For this review, take the finished solid that the model builds, in its own axes (mm). A direction names the side the tool comes from. Round coordinates to 2 decimals unless told otherwise and drop trailing zeros.
from build123d import *

# Parameters (mm, degrees)
BOSS_EXTRUDE1_DEPTH   = 12.7
KES_EKSTR_ZYON1_DEPTH = 22.86
SKETCH3_W             = 3.175
SKETCH3_H             = 4.501579944
KES_EKSTR_ZYON2_DEPTH = 22.86
KES_EKSTR_ZYON3_DEPTH = 22.86
KES_EKSTR_ZYON4_DEPTH = 11.43
RADYUS1_R             = 2.032
RADYUS2_R             = 1.27
IZIM2_W               = 3.81
IZIM2_H               = 25.4
KES_EKSTR_ZYON5_DEPTH = 22.86
IZIM3_W               = 8.451203014
IZIM3_H               = 0.1524
KES_EKSTR_ZYON6_DEPTH = 22.86
KES_EKSTR_ZYON7_DEPTH = 22.86
KES_EKSTR_ZYON8_DEPTH = 22.86
RADYUS3_R             = 0.254


with BuildPart() as part:
    # Sketch1 → Boss-Extrude1 (new, symmetric)
    with BuildSketch(Plane.XY):
        Polygon((-3.96875, 0), (3.96875, 0), (3.175, 4.501579944), (6.35, 4.501579944), (6.35, 55.301579944), (-6.35, 55.301579944), (-6.35, 4.501579944), (-3.175, 4.501579944), align=None)
    extrude(amount=BOSS_EXTRUDE1_DEPTH, both=True)

    # Sketch2 → Kes-Ekstrüzyon1 (cut)
    with BuildSketch(Plane(origin=(6.35, 0, 0), x_dir=(0, 0, -1), z_dir=(1, 0, 0))):
        with BuildLine():
            Line((9.525, 55.301579944), (-12.7, 55.301579944))
            Line((-12.7, 55.301579944), (-12.7, 10.851579944))
            ThreePointArc((-12.7, 10.851579944), (-6.8341108, 35.699885344), (9.525, 55.301579944))
        make_face()
    extrude(amount=-KES_EKSTR_ZYON1_DEPTH, mode=Mode.SUBTRACT)

    # Sketch3 → Kes-Ekstrüzyon2 (cut)
    with BuildSketch(Plane(origin=(6.35, 0, 0), x_dir=(0, 0, -1), z_dir=(1, 0, 0))):
        with Locations((11.1125, 2.250789972)):
            Rectangle(SKETCH3_W, SKETCH3_H)
    extrude(amount=-KES_EKSTR_ZYON2_DEPTH, mode=Mode.SUBTRACT)

    # Sketch4 → Kes-Ekstrüzyon3 (cut)
    with BuildSketch(Plane(origin=(6.35, 0, 0), x_dir=(0, 0, -1), z_dir=(1, 0, 0))):
        with BuildLine():
            Line((12.7, 52.126579944), (12.7, 4.501579944))
            ThreePointArc((12.7, 4.501579944), (6.35, 28.314079944), (12.7, 52.126579944))
        make_face()
    extrude(amount=-KES_EKSTR_ZYON3_DEPTH, mode=Mode.SUBTRACT)

    # Çizim1 → Kes-Ekstrüzyon4 (cut, symmetric)
    with BuildSketch(Plane(origin=(0, 0, 0), x_dir=(0, 0, -1), z_dir=(1, 0, 0))):
        with BuildLine():
            Line((-8.89, 10.851579944), (-8.89, 7.041579944))
            ThreePointArc((-8.89, 7.041579944), (-0.463388354, 8.480106364), (7.963223293, 7.041579944))
            ThreePointArc((7.963223293, 7.041579944), (3.304329022, 27.827298707), (7.564597424, 48.698367522))
            ThreePointArc((7.564597424, 48.698367522), (-4.598410017, 31.486096575), (-8.89, 10.851579944))
        make_face()
    extrude(amount=KES_EKSTR_ZYON4_DEPTH, both=True, mode=Mode.SUBTRACT)

    # Radyus1
    radyus1_edges = [part.edges().sort_by_distance(p)[0] for p in [
        (0, 7.041579944, -7.963223293),
        (0, 7.041579944, 8.89),
    ]]
    fillet(radyus1_edges, radius=RADYUS1_R)

    # Radyus2
    radyus2_edges = [part.edges().sort_by_distance(p)[0] for p in [
        (0, 48.698367522, -7.564597424),
    ]]
    fillet(radyus2_edges, radius=RADYUS2_R)

    # Çizim2 → Kes-Ekstrüzyon5 (cut)
    with BuildSketch(Plane.XY.offset(-2.54)):
        with Locations((0, 25.4)):
            Rectangle(IZIM2_W, IZIM2_H)
    extrude(amount=-KES_EKSTR_ZYON5_DEPTH, mode=Mode.SUBTRACT)

    # Çizim3 → Kes-Ekstrüzyon6 (cut)
    with BuildSketch(Plane(origin=(0, 0, -9.525), x_dir=(-1, 0, 0), z_dir=(0, 0, -1))):
        Rectangle(IZIM3_W, IZIM3_H)
    extrude(amount=-KES_EKSTR_ZYON6_DEPTH, mode=Mode.SUBTRACT)

    # Çizim4 → Kes-Ekstrüzyon7 (cut)
    with BuildSketch(Plane(origin=(0, 0, -9.525), x_dir=(-1, 0, 0), z_dir=(0, 0, -1))):
        Polygon((3.149208164, 4.501579944), (3.943735883, -0.004410664), (3.96875, 0), (3.175, 4.501579944), align=None)
        Polygon((-3.943735883, -0.004410664), (-3.149985883, 4.497169281), (-3.149208164, 4.501579944), (-3.175, 4.501579944), (-3.96875, 0), align=None)
    extrude(amount=-KES_EKSTR_ZYON7_DEPTH, mode=Mode.SUBTRACT)

    # Çizim7 → Kes-Ekstrüzyon8 (cut)
    with BuildSketch(Plane(origin=(0, 23.270981508, 23.270981508), x_dir=(-1, 0, 0), z_dir=(0, 0.7071067811865464, 0.7071067811865488))):
        Polygon((2.349914846, -48.08437831), (8.542960799, -39.080976931), (8.542960799, -48.08437831), align=None)
        Polygon((-8.542960799, -48.08437831), (-2.349914846, -48.08437831), (-8.542960799, -39.080976931), align=None)
    extrude(amount=-KES_EKSTR_ZYON8_DEPTH, mode=Mode.SUBTRACT)

    # Radyus3
    radyus3_edges = [part.edges().sort_by_distance(p)[0] for p in [
        (6.35, 7.676579944, 12.7),
        (0, 55.301579944, -9.525),
        (-5.120609971, 54.200188902, -8.104917983),
        (5.120609971, 54.200188902, -8.104917983),
        (-6.35, 7.676579944, 12.7),
        (-6.35, 34.080615313, 7.611288466),
        (6.35, 34.080615313, 7.611288466),
    ]]
    fillet(radyus3_edges, radius=RADYUS3_R)


solid = part.part
(1) For faces 5 (the face through (0.085, 35.339, 7.013)), 6 (the face through (1.905, 25, -5)), 7 (the face through (0, 54, -12.7)), 8 (the face through (0.089, 28.839, 5.664)), 9 (the face through (0, 2, -9.525)), list the 3-axis set-ups (+Z, -Z, +X, -X, +Y, -Y) from which the entire face can be reached by the end or side of a thin tool; tool diameter is ignored.
Geometry check:
face 5: +Z, +X, -X, +Y
face 6: -Z
face 7: -Z, +X, -X, +Y, -Y
face 8: +X, -X
face 9: -Z, +X, -X, -Y
(2) For line 1 along Z through (x, y) = (3, 39); line 2 along Z through (x, y) = (1.5, 41); line 3 along Y through (x, z) = (1, -0.75), list the stretches that pass through material, from the lowest coordinate up.
Geometry check:
line 1: z = -7.56 to -4.44, 0.57 to 5.04
line 2: z = -8.06 to -4.91, -0.8 to 3.81
line 3: y = 0.08 to 8.45, 40.93 to 47.1
(3) We need section A-A, the plane y = 18. State how many separate pieces and enclosed holes the cut face has, and give its area (3 significant figures).
Geometry check:
separate pieces: 3
enclosed holes: 0
area: 76.5 mm2
(4) For pin 1 Ø0.5 at (x, y) = (-2, 10.5) entering from -Z; pin 2 Ø3 at (x, z) = (-1.5, -4.5) entering from +Y (3 decimals); pin 3 Ø1.6 at (x, z) = (-0.5, -7) entering from +Y, all flat-tipped, find the tip position at first contact; note any pin that passes through.
Geometry check:
pin 1: stops at z = -9.89
pin 2: stops at y = 52.425
pin 3: stops at y = 53.95
(5) Mouldability with a two-part tool opening along X and no side actions: class faces 1 (the face through (-3.534, 2.32, 1.432)), 2 (the face through (0, 12.7, -7)), 3 (the face through (0.09, 8.18, 8.14)), 4 (the face through (6.35, 23, -4)) as pulls with the +X half, pulls with the -X half, needs draft (parallel to the pull), parting line crosses it, or undercut.
Geometry check:
face 1: pulls with the -X half
face 2: undercut
face 3: needs draft
face 4: pulls with the +X half
